Geometry check sheet. Reference: the model listing, model coordinates, mm. Face numbers are marked on the shaded views. A direction names the side the tool comes from. Round coordinates to 2 decimals unless told otherwise and drop trailing zeros. Order: outer loops, then holes, each group sorted by start corner. A loop starts at its lowest first (then second) coordinate and runs counter-clockwise, first axis right, second up.
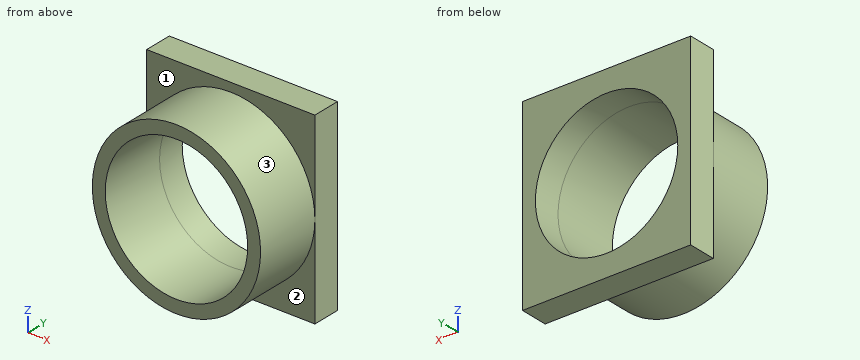
```python
from build123d import *

# Parameters (mm, degrees)
F0_W     = 30
F0_H     = 33.1
F1_DEPTH = 5
F2_R     = 15
F2_R_2   = 12.7
F3_DEPTH = 12
F4_R     = 12.7
F5_DEPTH = 25


with BuildPart() as f1:
    # F0 (on Front) → F1 (new body)
    with BuildSketch(Plane.XZ):
        Rectangle(F0_W, F0_H)
    extrude(amount=F1_DEPTH)

    # F2 (on face) → F3 (join)
    with BuildSketch(Plane.XZ.offset(5)):
        Circle(F2_R)
        Circle(F2_R_2, mode=Mode.SUBTRACT)
    extrude(amount=F3_DEPTH)

    # F4 (on face) → F5 (cut)
    with BuildSketch(Plane.XZ.offset(5)):
        Circle(F4_R)
    extrude(amount=-F5_DEPTH, mode=Mode.SUBTRACT)


solid = f1.part
```
(1) Sectioned sample at C-C, the plane y = -7.25. Record the cut outline in (x, z), and give its area (3 significant figures).
Returned:
outline: circle Ø30 at (0, 0); hole circle Ø25.4 at (0, 0)
area: 200 mm2
(2) Set-up check for the marked faces 1, 2 and 3: record each of +Z, -Z, +X, -X, +Y, -Y from which the full face is reachable in a straight line by a thin tool's end or side.
Returned:
face 1: +Z, -Y
face 2: -Z, -Y
face 3: -Y
(3) Sectioned sample at B-B, the plane z = -10. Record the cut outline in (x, y), and give its area (3 significant figures).
Returned:
outline: (-15, -5) - (-11.18, -5) - (-11.18, -17) - (-7.83, -17) - (-7.83, 0) - (-15, 0) - close; (7.83, -17) - (11.18, -17) - (11.18, -5) - (15, -5) - (15, 0) - (7.83, 0) - close
area: 152 mm2
(4) Depth check by flat-ended pin: P1, Ø1, axis at x = -3, y = -7.5, coming from the +Z side; P2, Ø18, axis at x = -2, z = 7, coming from the -Y side; P3, Ø5, axis at x = 1, z = -9.5, coming from the -Y side; P4, Ø4, axis at y = -9.5, z = 6.5, coming from the +X side. Enter the tip coordinate at first touch or a pass-through.
Returned:
P1: stops at z = 14.79
P2: stops at y = -17
P3: passes through
P4: stops at x = 14.31
(5) Sectioned sample at A-A, the plane x = 0. Record the cut outline in (y, z), and give its area (3 significant figures).
Returned:
outline: (-17, -15) - (-5, -15) - (-5, -16.55) - (0, -16.55) - (0, -12.7) - (-17, -12.7) - close; (-17, 12.7) - (0, 12.7) - (0, 16.55) - (-5, 16.55) - (-5, 15) - (-17, 15) - close
area: 93.7 mm2
(6) Material ranges on line 1 (Z direction, x = 0, y = -2.6); line 2 (Z direction, x = 0, y = -7.5); line 3 (X direction, y = -7, z = 4), recorded low to high.
Returned:
line 1: z = -16.55 to -12.7, 12.7 to 16.55
line 2: z = -15 to -12.7, 12.7 to 15
line 3: x = -14.46 to -12.05, 12.05 to 14.46
